Here's how the part is built. I have some questions about the finished solid (model axes, mm). Round coordinates to 2 decimals unless told otherwise and drop trailing zeros. Order: outer loops, then holes, each group sorted by start corner. A loop starts at its lowest first (then second) coordinate and runs counter-clockwise, first axis right, second up.
```python
from build123d import *

# Parameters (mm, degrees)
SKETCH1_W           = 38
SKETCH1_H           = 38
SKETCH1_R           = 1
SKETCH1_W_2         = 9
SKETCH1_H_2         = 1.2
SKETCH1_W_3         = 1.2
SKETCH1_H_3         = 9
BOSS_EXTRUDE1_DEPTH = 1.6


with BuildPart() as part:
    # Sketch1 → Boss-Extrude1 (new body)
    with BuildSketch(Plane.XZ):
        Rectangle(SKETCH1_W, SKETCH1_H)
        with Locations(Location((-14, -14, 0), (0, 0, 90))):
            Circle(SKETCH1_R, mode=Mode.SUBTRACT)
        with Locations(Location((-14, 14, 0), (0, 0, 90))):
            Circle(SKETCH1_R, mode=Mode.SUBTRACT)
        with Locations(Location((14, -14, 0), (0, 0, 90))):
            Circle(SKETCH1_R, mode=Mode.SUBTRACT)
        with Locations(Location((14, 14, 0), (0, 0, 90))):
            Circle(SKETCH1_R, mode=Mode.SUBTRACT)
        with BuildLine():
            Line((6.5, 17.2), (16.2, 17.2))
            ThreePointArc((16.2, 17.2), (17.907106781, 17.907106781), (17.2, 16.2))
            Line((17.2, 16.2), (17.2, 6.5))
            Line((17.2, 6.5), (16, 6.5))
            Line((16, 6.5), (16, 16))
            Line((16, 16), (6.5, 16))
            Line((6.5, 16), (6.5, 17.2))
        make_face(mode=Mode.SUBTRACT)
        with BuildLine():
            Line((-6.5, -17.2), (-16.2, -17.2))
            ThreePointArc((-16.2, -17.2), (-17.907106781, -17.907106781), (-17.2, -16.2))
            Line((-17.2, -16.2), (-17.2, -6.5))
            Line((-17.2, -6.5), (-16, -6.5))
            Line((-16, -6.5), (-16, -16))
            Line((-16, -16), (-6.5, -16))
            Line((-6.5, -16), (-6.5, -17.2))
        make_face(mode=Mode.SUBTRACT)
        with Locations((0, 16.6)):
            Rectangle(SKETCH1_W_2, SKETCH1_H_2, mode=Mode.SUBTRACT)
        with BuildLine():
            Line((6.5, -16), (16, -16))
            Line((16, -16), (16, -6.5))
            Line((16, -6.5), (17.2, -6.5))
            Line((17.2, -6.5), (17.2, -16.2))
            ThreePointArc((17.2, -16.2), (17.907106781, -17.907106781), (16.2, -17.2))
            Line((16.2, -17.2), (6.5, -17.2))
            Line((6.5, -17.2), (6.5, -16))
        make_face(mode=Mode.SUBTRACT)
        with Locations((-16.6, 0)):
            Rectangle(SKETCH1_W_3, SKETCH1_H_3, mode=Mode.SUBTRACT)
        with Locations((16.6, 0)):
            Rectangle(SKETCH1_W_3, SKETCH1_H_3, mode=Mode.SUBTRACT)
        with BuildLine():
            Line((-16, 16), (-16, 6.5))
            Line((-16, 6.5), (-17.2, 6.5))
            Line((-17.2, 6.5), (-17.2, 16.2))
            ThreePointArc((-17.2, 16.2), (-17.907106781, 17.907106781), (-16.2, 17.2))
            Line((-16.2, 17.2), (-6.5, 17.2))
            Line((-6.5, 17.2), (-6.5, 16))
            Line((-6.5, 16), (-16, 16))
        make_face(mode=Mode.SUBTRACT)
        with Locations((0, -16.6)):
            Rectangle(SKETCH1_W_2, SKETCH1_H_2, mode=Mode.SUBTRACT)
    extrude(amount=-BOSS_EXTRUDE1_DEPTH)


solid = part.part
```
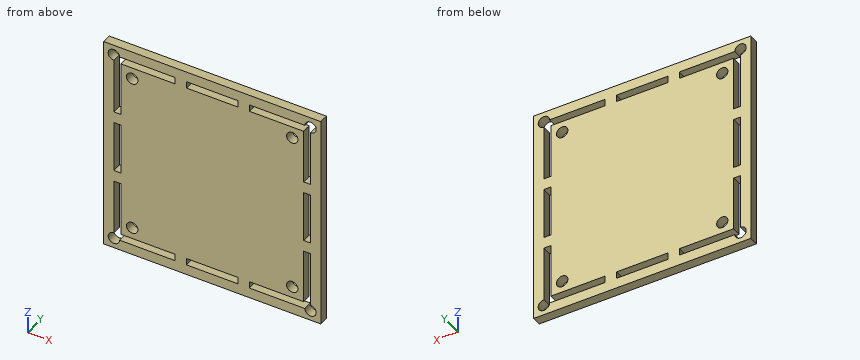
1) If we section it at B-B (x = -7): Write out the boundary of the cut face in (y, z).
2) If we section it at D-D (z = -12.5): Write out the boundary of the cut face in (x, y).
3) I need wall thicknesses on line 1 (Z direction, x = 2.5, y = 1.15); line 2 (Z direction, x = -14, y = 0.95). Which ranges of each line are inside material? Lowest first, please.
4) If we section it at C-C (x = -14): Write out the boundary of the cut face in (y, z).
5) If we section it at A-A (z = 14): Write out the boundary of the cut face in (x, y), plus the area to 3 significant figures.
Solutions:
1. outline: (0, -19) - (1.6, -19) - (1.6, -17.2) - (0, -17.2) - close; (0, -16) - (1.6, -16) - (1.6, 16) - (0, 16) - close; (0, 17.2) - (1.6, 17.2) - (1.6, 19) - (0, 19) - close
2. outline: (-19, 0) - (-17.2, 0) - (-17.2, 1.6) - (-19, 1.6) - close; (-16, 0) - (16, 0) - (16, 1.6) - (-16, 1.6) - close; (17.2, 0) - (19, 0) - (19, 1.6) - (17.2, 1.6) - close
3. line 1: z = -19 to -17.2, -16 to 16, 17.2 to 19
3. line 2: z = -19 to -17.2, -16 to -15, -13 to 13, 15 to 16, 17.2 to 19
4. outline: (0, -19) - (1.6, -19) - (1.6, -17.2) - (0, -17.2) - close; (0, -16) - (1.6, -16) - (1.6, -15) - (0, -15) - close; (0, -13) - (1.6, -13) - (1.6, 13) - (0, 13) - close; (0, 15) - (1.6, 15) - (1.6, 16) - (0, 16) - close; (0, 17.2) - (1.6, 17.2) - (1.6, 19) - (0, 19) - close
5. outline: (-19, 0) - (-17.2, 0) - (-17.2, 1.6) - (-19, 1.6) - close; (-16, 0) - (-15, 0) - (-15, 1.6) - (-16, 1.6) - close; (-13, 0) - (13, 0) - (13, 1.6) - (-13, 1.6) - close; (15, 0) - (16, 0) - (16, 1.6) - (15, 1.6) - close; (17.2, 0) - (19, 0) - (19, 1.6) - (17.2, 1.6) - close
5. area: 50.6 mm2
